from build123d import *

# Parameters (mm, degrees)
SKETCH2_R           = 17
BOSS_EXTRUDE1_DEPTH = 12
SKETCH3_R           = 16.15
SKETCH3_R_2         = 10
CUT_EXTRUDE1_DEPTH  = 8
FILLET1_R           = 1
SKETCH4_W           = 8.2
SKETCH4_H           = 3.2
CUT_EXTRUDE2_DEPTH  = 27.870057685


with BuildPart() as part:
    # Sketch2 → Boss-Extrude1 (new body)
    with BuildSketch(Plane.XY):
        Circle(SKETCH2_R)
    extrude(amount=BOSS_EXTRUDE1_DEPTH)

    # Sketch3 → Cut-Extrude1 (cut)
    # profile 1 of 2: a face of its own
    with BuildSketch(Plane.XY.offset(12)):
        Circle(SKETCH3_R)
        Circle(SKETCH3_R_2, mode=Mode.SUBTRACT)
    # profile 2 of 2: a face of its own
    with BuildSketch(Plane.XY.offset(12)):
        Circle(SKETCH3_R_2)
    extrude(amount=-CUT_EXTRUDE1_DEPTH, mode=Mode.SUBTRACT)

    # Fillet1
    fillet1_edges = [part.edges().sort_by_distance(p)[0] for p in [
        (-16.15, 0, 4),
    ]]
    fillet(fillet1_edges, radius=FILLET1_R)

    # Sketch4 → Cut-Extrude2 (cut, through all)
    with BuildSketch(Plane(origin=(0, 0, 0), x_dir=(-1, 0, 0), z_dir=(0, 0, -1))):
        with Locations((0, 6.312686907)):
            Rectangle(SKETCH4_W, SKETCH4_H)
        with BuildLine():
            Line((2.925, -5.786814383), (-2.925, -5.786814383))
            ThreePointArc((-2.925, -5.786814383), (-4.65, -4.061814383), (-2.925, -2.336814383))
            Line((-2.925, -2.336814383), (2.925, -2.336814383))
            ThreePointArc((2.925, -2.336814383), (4.65, -4.061814383), (2.925, -5.786814383))
        make_face()
    extrude(amount=-CUT_EXTRUDE2_DEPTH, mode=Mode.SUBTRACT)


solid = part.part
Geometry: final body of the model. Coordinates: model frame, mm. A direction names the side the tool comes from. Coordinates: 2 decimals unless noted, no trailing zeros. Order: outer loops, then holes, each group sorted by start corner. A loop starts at its lowest first (then second) coordinate and runs counter-clockwise, first axis right, second up.
(1) Section query A-A (x = 0). Return the cut outline in (y, z), plus the area to 3 significant figures.
(2) Draft query along Y for faces 4 (the face through (0, -5.787, 2)), 5 (the face through (0, 0, 4)), 6 (the face through (9.139, 14.334, 5.916)), 7 (the face through (0, 0, 0)). Return one class per face: pulls with the +Y half, pulls with the -Y half, needs draft (parallel to the pull), parting line crosses it, or undercut.
(3) Section query C-C (y = 0). Return the cut outline in (x, z).
(4) Material intervals for probe 1 along Y at (x, z) = (0, 9.5); probe 2 along Y at (x, z) = (-0.5, 0.5); probe 3 along Z at (x, y) = (-12.5, -7), sorted ascending.
(5) First-contact query: pin 1 (6 mm diameter, centred on y = 12, z = 2, fed in from -X); pin 2 (2 mm diameter, centred on y = 7.5, z = 6.5, fed in from +X); pin 3 (15 mm diameter, centred on x = -4.5, y = 2.5, fed in from +Z). Flat tips, straight axial feed; report the tip coordinate or a pass-through.
(6) Section query D-D (z = 4.5). Return the cut outline in (x, y), plus the area to 3 significant figures.
(7) Section query B-B (z = 10). Return the cut outline in (x, y), plus the area to 3 significant figures.
(8) Access query for faces 1 (the face through (-3.501, -15.766, 8.549)), 2 (the face through (9, -14, 12)), 3 (the face through (-4.65, -4.02, 1.97)). Directions: +Z, -Z, +X, -X, +Y, -Y. A direction counts if a zero-diameter tool reaches every point of the face in a straight line with its end or side. Return the directions, or none.
Solution:
1. outline: (-17, 0) - (-5.79, 0) - (-5.79, 4) - (-15.15, 4) arc R1 cw to (-16.15, 5) - (-16.15, 12) - (-17, 12) - close; (-2.34, 0) - (4.71, 0) - (4.71, 4) - (-2.34, 4) - close; (7.91, 0) - (17, 0) - (17, 12) - (16.15, 12) - (16.15, 5) arc R1 cw to (15.15, 4) - (7.91, 4) - close
1. area: 123 mm2
2. face 4: undercut
2. face 5: undercut
2. face 6: parting line crosses it
2. face 7: needs draft
3. outline: (-17, 0) - (17, 0) - (17, 12) - (16.15, 12) - (16.15, 5) arc R1 cw to (15.15, 4) - (-15.15, 4) arc R1 cw to (-16.15, 5) - (-16.15, 12) - (-17, 12) - close
4. probe 1: y = -17 to -16.15, 16.15 to 17
4. probe 2: y = -16.99 to -5.79, -2.34 to 4.71, 7.91 to 16.99
4. probe 3: z = 0 to 4
5. pin 1: stops at x = -14.42
5. pin 2: stops at x = 15.71
5. pin 3: stops at z = 4
6. outline: circle Ø34 at (0, 0); hole circle Ø32.03 at (0, 0)
6. area: 102 mm2
7. outline: circle Ø34 at (0, 0); hole circle Ø32.3 at (0, 0)
7. area: 88.5 mm2
8. face 1: +Z
8. face 2: +Z, +X, -X, +Y, -Y
8. face 3: +Z, -Z
